The listing builds one solid part. Answer for the finished solid, in the listing's coordinates (mm). A direction names the side the tool comes from. Round coordinates to 2 decimals unless told otherwise and drop trailing zeros. Write each loop counter-clockwise with the first axis right and the second up, starting at its lowest first coordinate (ties: lowest second). Pieces come first, ordered by that corner, then holes.
Item 1: Find section A-A on z = -10.75. Give the vertices of the cut face in (x, y), then the cut area to 3 significant figures.
Item 2: Find the intervals of material crossed by probe 1 along Y at (x, z) = (37, -14); probe 2 along X at (y, z) = (155.5, -1); probe 3 along X at (y, z) = (286, -1.75), in increasing order.
Item 3: Each of these flat-tipped pins is pushed along its axis until it touches: pin 1 (4 mm diameter, centred on x = 27.5, z = -17, fed in from -Y); pin 2 (11 mm diameter, centred on y = 289.5, z = -9.5, fed in from +X); pin 3 (4 mm diameter, centred on x = 23.5, z = -10, fed in from +Y). Where does it stop, or does it pass through?
Item 4: Find section B-B on x = 41. Give the vertices of the cut face in (y, z), then the cut area to 3 significant figures.
Item 5: A tool of negligible diameter and unlimited length cuts with its end or side. For faces 1 (the face through (0, 290, -10)), 2 (the face through (-113.594, 287.972, -10.098)), 3 (the face through (0, 10, -10)), from which of +Z, -Z, +X, -X, +Y, -Y can it reach the whole face along a straight path? Write none if from no direction.
```python
from build123d import *

# Parameters (mm, degrees)
F1_W     = 250
F1_H     = 300
F2_DEPTH = 20
F3_DEPTH = 18
F4_W     = 125
F4_H     = 20
F5_DEPTH = 18
F6_R     = 40
F7_R     = 3


with BuildPart() as f2:
    # F1 (on Top) → F2 (new body)
    with BuildSketch(Plane.XY):
        with Locations((0, 150)):
            Rectangle(F1_W, F1_H)
    extrude(amount=-F2_DEPTH)

    # F0 (on Front) → F3 (cut)
    with BuildSketch(Plane.XZ):
        with BuildLine():
            ThreePointArc((160.7967353507, 4.0303440201), (159.065909211, 1.1368225578), (155.8916596855, 0))
            Line((155.8916596855, 0), (45.0975336134, 0))
            Line((45.0975336134, 0), (45.0975336134, -5))
            Line((45.0975336134, -5), (0, -5))
            Line((0, -5), (0, -20.7676107392))
            ThreePointArc((0, -20.7676107392), (2.6525588341, -27.5510544306), (9.2030216628, -30.7358014241))
            Line((9.2030216628, -30.7358014241), (175.0106296305, -43.9924771707))
            ThreePointArc((175.0106296305, -43.9924771707), (194.4976732451, -37.7783808724), (204.0363591727, -19.684919832))
            Line((204.0363591727, -19.684919832), (219.923475276, 144.1129544091))
            ThreePointArc((219.923475276, 144.1129544091), (217.690858581, 151.4337512548), (210.9355750829, 155.0316379433))
            Line((210.9355750829, 155.0316379433), (195.5381857284, 156.525064604))
            ThreePointArc((195.5381857284, 156.525064604), (192.0716412109, 155.5604813638), (190.150414228, 152.518074652))
            Line((190.150414228, 152.518074652), (160.7967353507, 4.0303440201))
        make_face()
        with BuildLine():
            Line((45.0975336134, -5), (45.0975336134, 0))
            Line((45.0975336134, 0), (5, 0))
            ThreePointArc((5, 0), (1.4644660941, -1.4644660941), (0, -5))
            Line((0, -5), (45.0975336134, -5))
        make_face()
        with BuildLine():
            Line((5, 0), (45.0975336134, 0))
            Line((45.0975336134, 0), (45.0975336134, 7.6496871188))
            Line((45.0975336134, 7.6496871188), (0, 7.6496871188))
            Line((0, 7.6496871188), (0, -5))
            ThreePointArc((0, -5), (1.4644660941, -1.4644660941), (5, 0))
        make_face()
    extrude(amount=-F3_DEPTH, mode=Mode.SUBTRACT)

    # F4 (on face) → F5 (cut)
    with BuildSketch(Plane(origin=(0, 300, 0), x_dir=(-1, 0, 0), z_dir=(0, 1, 0))):
        with Locations((-62.5, -10)):
            Rectangle(F4_W, F4_H)
    extrude(amount=-F5_DEPTH, mode=Mode.SUBTRACT)

    # F6
    f6_edges = [f2.edges().sort_by_distance(p)[0] for p in [
        (-125, 300, -10),
        (-125, 0, -10),
        (125, 282, -10),
        (125, 18, -10),
    ]]
    fillet(f6_edges, radius=F6_R)

    # F7
    f7_edges = [f2.edges().sort_by_distance(p)[0] for p in [
        (0, 0, -10),
        (0, 300, -10),
        (42.5, 282, 0),
        (113.284271, 270.284271, 0),
        (0, 291, 0),
        (125, 150, 0),
        (-42.5, 300, 0),
        (113.284271, 29.715729, 0),
        (-113.284271, 288.284271, 0),
        (42.5, 18, 0),
        (-125, 150, 0),
        (0, 9, 0),
        (-113.284271, 11.715729, 0),
        (-42.5, 0, 0),
        (42.5, 282, -20),
        (113.284271, 270.284271, -20),
        (0, 291, -20),
        (125, 150, -20),
        (-42.5, 300, -20),
        (113.284271, 29.715729, -20),
        (-113.284271, 288.284271, -20),
        (42.5, 18, -20),
        (-125, 150, -20),
        (0, 9, -20),
        (-113.284271, 11.715729, -20),
        (-42.5, 0, -20),
    ]]
    fillet(f7_edges, radius=F7_R)


solid = f2.part
```
Check values:
1. outline: (-125, 40) arc R40 ccw to (-85, 0) - (-3, 0) arc R3 ccw to (0, 3) - (0, 18) - (85, 18) arc R40 ccw to (125, 58) - (125, 242) arc R40 ccw to (85, 282) - (0, 282) - (0, 297) arc R3 ccw to (-3, 300) - (-85, 300) arc R40 ccw to (-125, 260) - close
1. area: 69,100 mm2
2. probe 1: y = 18 to 282
2. probe 2: x = -124.24 to 124.24
2. probe 3: x = -115.04 to -0.27
3. pin 1: stops at y = 18
3. pin 2: stops at x = 0
3. pin 3: stops at y = 282
4. outline: (18, -17) arc R3 ccw to (21, -20) - (279, -20) arc R3 ccw to (282, -17) - (282, -3) arc R3 ccw to (279, 0) - (21, 0) arc R3 ccw to (18, -3) - close
4. area: 5,270 mm2
5. face 1: +Z, -Z, +X, +Y
5. face 2: +Z, -Z, -X, +Y
5. face 3: +Z, -Z, +X, -Y
